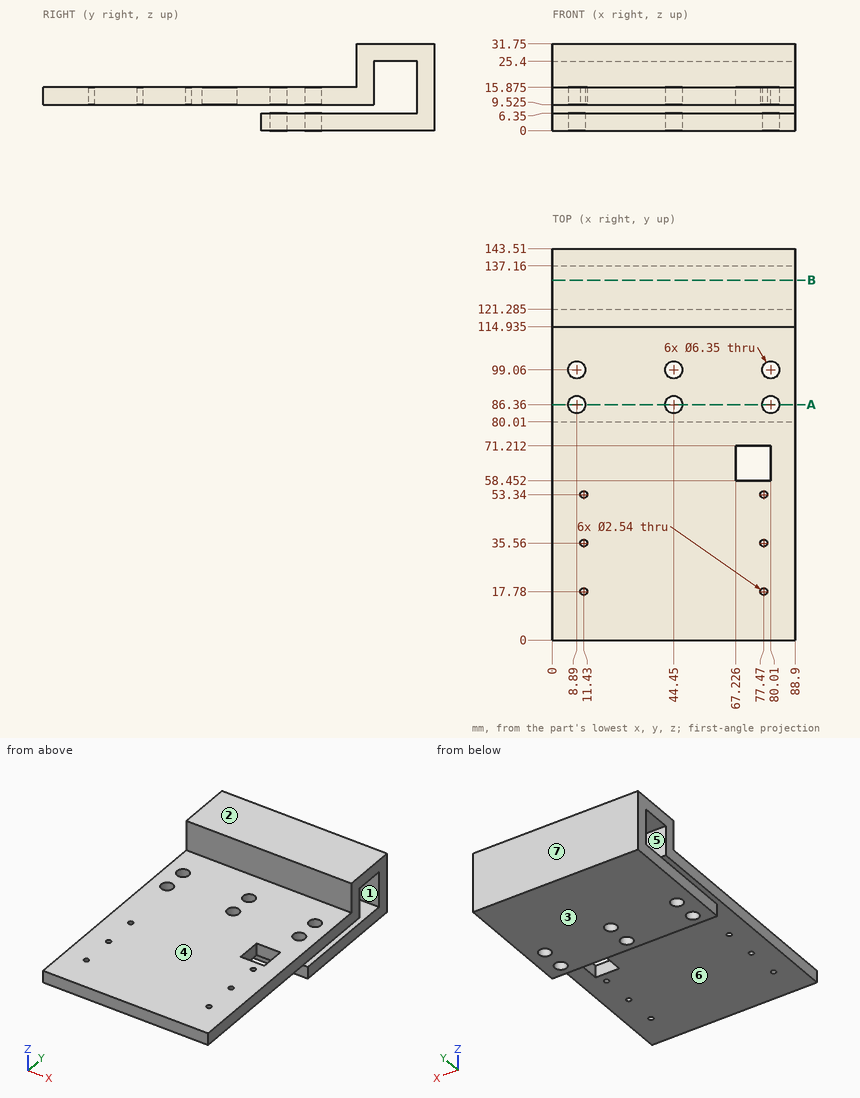
Here's the drawing with two shaded views (mm, measured from the low corner). I have some questions. A direction names the side the tool comes from. Coordinates: 2 decimals unless noted, no trailing zeros. Order: outer loops, then holes, each group sorted by start corner. A loop starts at its lowest first (then second) coordinate and runs counter-clockwise, first axis right, second up. Notation, with made-up numbers: (72, -2) -> (118, -2) arc R30 cw to (118, 30) -> close; hole circle Ø7 at (56.5, -23.5). An arc over 180 degrees is marked (long way). One line per question, with ' | ' between items.
Q1. If I drill on L1, parallel to X at y = 99.06, z = 11 (1 decimal); L2, parallel to X at y = 86, z = 14 (1 decimal); L3, parallel to Y at x = 49.5, z = 17 (1 decimal), over which ranges is the centre line in solid material (lowest first)?
Return value:
L1: 0 to 5.7, 12.1 to 41.3, 47.6 to 76.8, 83.2 to 88.9 | L2: 0 to 5.7, 12 to 41.3, 47.6 to 76.9, 83.2 to 88.9 | L3: 114.9 to 121.3, 137.2 to 143.5
Q2. On a 3-axis mill with a long thin cutter (end or side, diameter ignored), from which of +Z, -Z, +X, -X, +Y, -Y can I reach the whole of each face in a straight line? I mean the marked faces 4, 5, 6 and 7. Say none if no direction works.
Return value:
face 4: +Z, +X, -X, -Y | face 5: +X, -X | face 6: +X, -X, -Y | face 7: +Z, -Z, +X, -X, +Y
Q3. Imagine slicing it at A-A on y = 86.36. State how many separate pieces and enclosed holes the cut face has, and give its area (3 significant figures).
Return value:
separate pieces: 8 | enclosed holes: 0 | area: 887 mm²
Q4. I'm going to push flat-ended pins straight in: P1, Ø3.5, axis at x = 77.47, y = 53.34, coming from the +Z side (3 decimals); P2, Ø1.5, axis at x = 77.47, y = 17.78, coming from the +Z side; P3, Ø1, axis at x = 55, z = 5.5, coming from the -Y side; P4, Ø1, axis at x = 77, y = 28.5, coming from the -Z side (3 decimals). Where does each tip first touch, or does it pass through?
Return value:
P1: z = 15.875 | P2: through | P3: y = 80.01 | P4: z = 9.525
Q5. Imagine slicing it at B-B on y = 132. Please give me the cut outline in (x, z).
Return value:
outline: (0, 0) -> (88.9, 0) -> (88.9, 6.35) -> (0, 6.35) -> close; (0, 25.4) -> (88.9, 25.4) -> (88.9, 31.75) -> (0, 31.75) -> close
Q6. Thinking about a two-plate mould opening in Z: for the marked faces 1, 2 and 3, which applies, pulls with the +Z half, pulls with the -Z half, needs draft (parallel to the pull), parting line crosses it, or undercut?
Return value:
face 1: undercut | face 2: pulls with the +Z half | face 3: pulls with the -Z half
